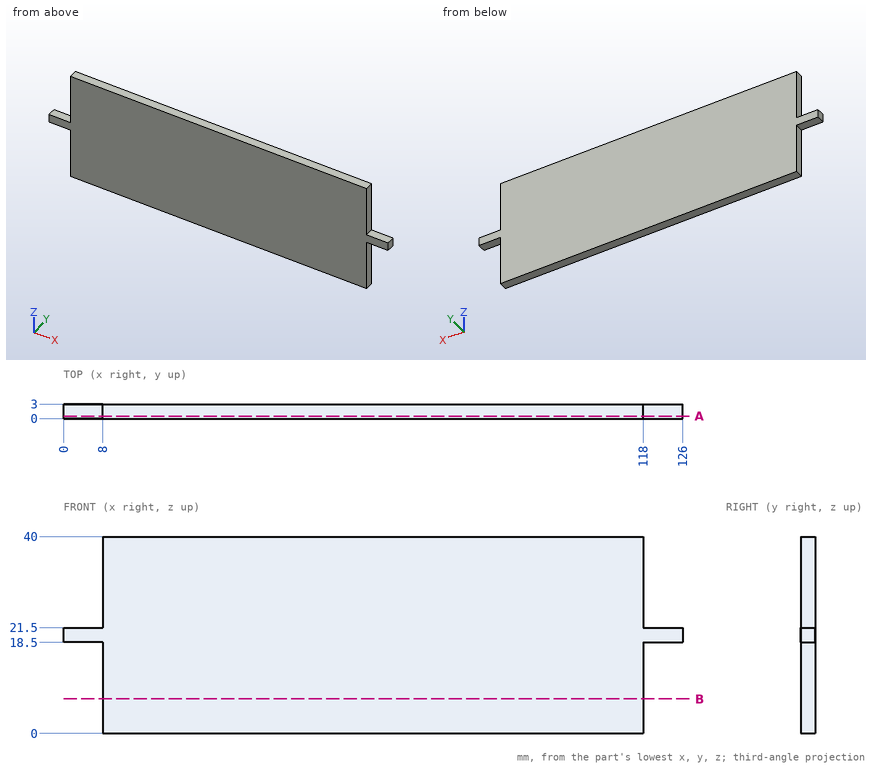
Verification items for this drawing (mm, ordinates from the low corner). Give positions to 0.01 mm unless a question says otherwise; leave off trailing zeros. Write each loop counter-clockwise with the first axis right and the second up, starting at its lowest first coordinate (ties: lowest second). Pieces come first, ordered by that corner, then holes. Notation, with made-up numbers: (18, -2) -> (63, -2) arc R22 ccw to (63, 7) -> close; hole circle Ø6 at (77.25, 64). An arc over 180 degrees is marked (long way). Use one line per item in the form item = value.
Item 1: Depth check by flat-ended pin: pin 1 Ø0.9 at (y, z) = (1.5, 10.5) entering from +X; pin 2 Ø1 at (x, y) = (101.5, 0.5) entering from -Z; pin 3 Ø1.5 at (y, z) = (1.5, 31) entering from -X; pin 4 Ø0.9 at (x, y) = (122.5, 1.5) entering from +Z. Enter the tip coordinate at first touch or a pass-through.
Results list:
pin_1 = 118
pin_2 = 0
pin_3 = 8
pin_4 = 21.5
Item 2: Sectioned sample at B-B on z = 7. Enter the section's corners in (x, y), plus the area to 3 significant figures.
Results list:
outline = (8, 0) -> (118, 0) -> (118, 3) -> (8, 3) -> close
area = 330 mm2
Item 3: Scan lines: line 1 (X direction, y = 1.7, z = 2); line 2 (Z direction, x = 7, y = 1.7). Record each from-to range of solid material in increasing order.
Results list:
line_1 = 8 to 118
line_2 = 18.5 to 21.5
Item 4: Sectioned sample at A-A on y = 0.55. Enter the section's corners in (x, z).
Results list:
outline = (0, 18.5) -> (8, 18.5) -> (8, 0) -> (118, 0) -> (118, 18.5) -> (126, 18.5) -> (126, 21.5) -> (118, 21.5) -> (118, 40) -> (8, 40) -> (8, 21.5) -> (0, 21.5) -> close
